The drawing under review shows one solid part. Ordinate dimensions are in mm from its lowest x, y, z. Give positions to 0.01 mm unless a question says otherwise; leave off trailing zeros. Loops run counter-clockwise (first coordinate to the right, second up) from the corner with the lowest first, then second, coordinate; pieces in that order, holes last. Notation, with made-up numbers: (-25.5, 82) - (-20.5, 82) arc R21 cw to (-20.5, 120) - close; hole circle Ø5 at (0.5, 77.25). An arc over 180 degrees is marked (long way). Return JSON: item names as keys, results as strings. Group by question number.
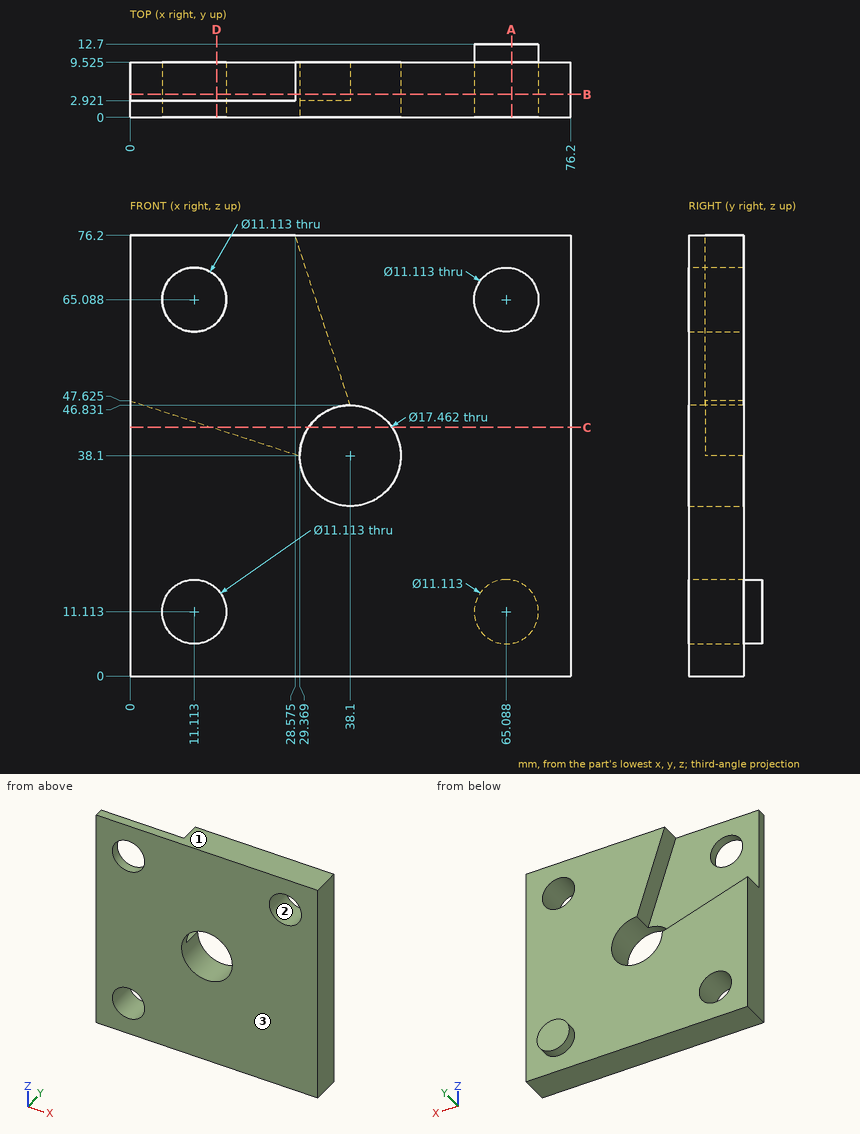
1) We need section A-A, the plane x = 66. Write out the cut boundary in (y, z) (1 decimal).
2) For pin 1 Ø23 at (x, z) = (37.5, 33) entering from +Y (1 decimal); pin 2 Ø4 at (x, z) = (29, 52.5) entering from +Y, all flat-tipped, find the tip position at first contact; note any pin that passes through.
3) We need section D-D, the plane x = 15. Write out the cut boundary in (y, z) (1 decimal), plus the area to 3 significant figures.
4) We need section C-C, the plane z = 43. Write out the cut boundary in (x, y) (1 decimal).
5) Draft analysis for pull direction Z (two halves, no side actions). For the marked faces 1, 2 and 3, state which applies: +Z half, -Z half, draft (parallel to the pull), parting line (faces both ways), or undercut.
6) To check wall thickness, follow line 1 (Z direction, x = 38.1, y = 2); line 2 (Z direction, x = 16, y = 1.5) (1 decimal); line 3 (Z direction, x = 13, y = 2.5) (1 decimal). State the ranges of each line that lie inside material, in increasing order.
7) We need section B-B, the plane y = 4. Write out the cut boundary in (x, z) (1 decimal), plus the area to 3 significant figures.
Findings:
{
 "1": {"outline": "(0, 0) - (9.5, 0) - (9.5, 5.6) - (12.7, 5.6) - (12.7, 16.6) - (9.5, 16.6) - (9.5, 59.6) - (0, 59.6) - close; (0, 70.6) - (9.5, 70.6) - (9.5, 76.2) - (0, 76.2) - close"},
 "2": {"pin 1": "stops at y = 9.5", "pin 2": "stops at y = 2.92"},
 "3": {"outline": "(0, 0) - (9.5, 0) - (9.5, 7.1) - (0, 7.1) - close; (0, 15.1) - (9.5, 15.1) - (9.5, 42.8) - (2.9, 42.8) - (2.9, 61.1) - (0, 61.1) - close; (0, 69.1) - (2.9, 69.1) - (2.9, 76.2) - (0, 76.2) - close", "area": "406 mm^2"},
 "4": {"outline": "(0, 0) - (30.9, 0) - (30.9, 2.9) - (14.3, 2.9) - (14.3, 9.5) - (0, 9.5) - close; (45.3, 0) - (76.2, 0) - (76.2, 9.5) - (45.3, 9.5) - close"},
 "5": {"face 1": "+Z half", "face 2": "undercut", "face 3": "draft"},
 "6": {"line 1": "z = 0 to 29.37, 46.83 to 76.2", "line 2": "z = 0 to 8.5, 13.8 to 62.4, 67.7 to 76.2", "line 3": "z = 0 to 5.9, 16.3 to 59.9, 70.3 to 76.2"},
 "7": {"outline": "(0, 0) - (76.2, 0) - (76.2, 76.2) - (28.6, 76.2) - (38.1, 46.8) arc R8.7 cw (long way) to (29.4, 38.1) - (0, 47.6) - close; hole circle Ø11.1 at (11.1, 11.1); hole circle Ø11.1 at (65.1, 65.1)", "area": "4,260 mm^2"}
}
